Print and shaded views of the part. All mm, measured from the part's lowest x, y and z. Give positions to 0.01 mm unless a question says otherwise; leave off trailing zeros. Order: outer loops, then holes, each group sorted by start corner. A loop starts at its lowest first (then second) coordinate and runs counter-clockwise, first axis right, second up. Notation, with made-up numbers: (-31, 14) -> (-9, 14) arc R4 cw to (-9, 19) -> close; hole circle Ø1 at (62, -12). An arc over 180 degrees is marked (long way). One line per question, with ' | ' between items. Start each with the question number.
(1) Cut at A-A (z = 1.9). Give the cut face in (x, y), then the cut area to 3 significant figures.
(2) Cut at B-B (x = 17.25). Give the cut face in (y, z) (3 decimals).
(3) Pull direction Z, two halves, no side cores. Call the marked faces 1, 2, 3 and 4: +Z half, -Z half, draft (parallel to the pull), parting line (faces both ways), or undercut.
(4) Cut at C-C (y = 17.75). Give the cut face in (x, z).
(5) Drill centre lines: L1, parallel to Y at x = 7.25, z = 1.1; L2, parallel to X at y = 16.5, z = 0.95; L3, parallel to X at y = 17.5, z = 1.45. Where is each one in solid material? Low to high. Write a range as from..to.
(6) Pin check, flat tips, straight feed: pin 1 Ø6 at (x, y) = (4, 10.5) entering from -Z; pin 2 Ø3 at (x, z) = (2.5, 4.5) entering from +Y; pin 3 Ø1 at (x, z) = (17.5, 4.5) entering from -Y. Stop position of each tip, or through.
(7) Cut at D-D (z = 0.3). Give the cut face in (x, y).
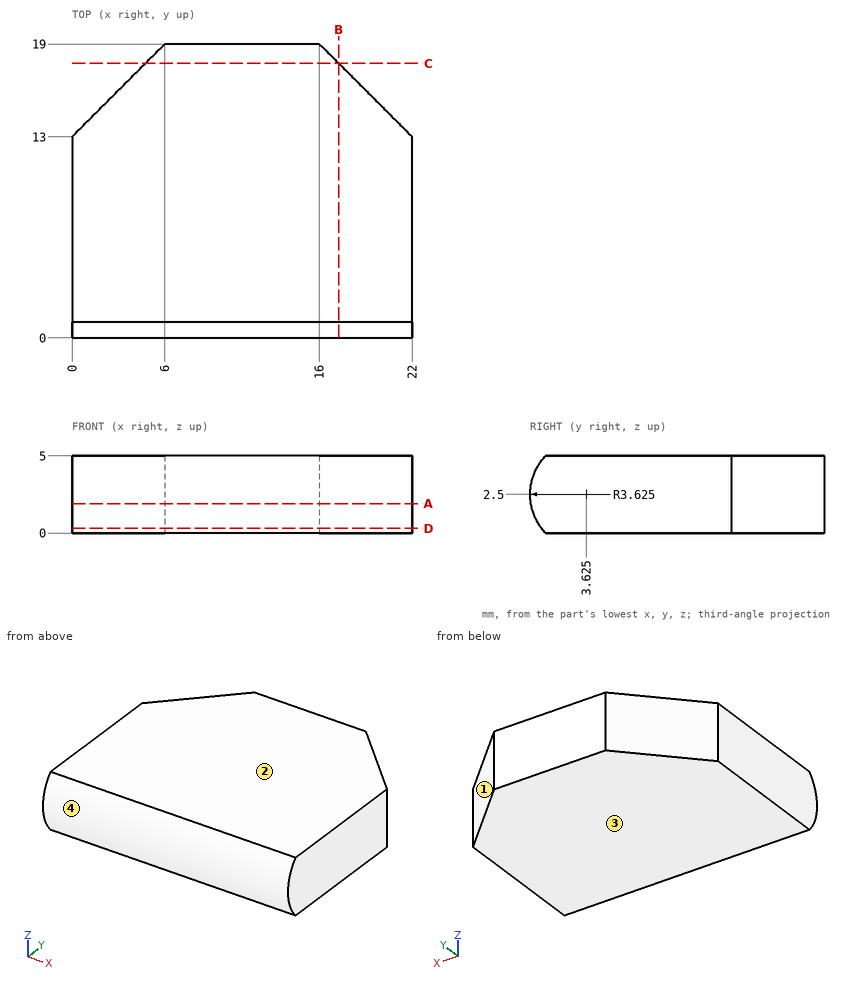
Result set:
1) outline: (0, 0.05) -> (22, 0.05) -> (22, 13) -> (16, 19) -> (6, 19) -> (0, 13) -> close | area: 381 mm2
2) outline: (1, 0) -> (17.75, 0) -> (17.75, 5) -> (1, 5) arc R3.625 ccw to start
3) face 1: draft | face 2: +Z half | face 3: -Z half | face 4: parting line
4) outline: (4.75, 0) -> (17.25, 0) -> (17.25, 5) -> (4.75, 5) -> close
5) L1: y = 0.28..19 | L2: x = 3.5..18.5 | L3: x = 4.5..17.5
6) pin 1: stops at z = 0 | pin 2: stops at y = 17 | pin 3: stops at y = 0.32
7) outline: (0, 0.74) -> (22, 0.74) -> (22, 13) -> (16, 19) -> (6, 19) -> (0, 13) -> close
